Can you work these out from the drawing? Everything is in mm from the part's minimum corner. Give positions to 0.01 mm unless a question says otherwise; leave off trailing zeros. Order: outer loops, then holes, each group sorted by start corner. A loop starts at its lowest first (then second) coordinate and runs counter-clockwise, first axis right, second up. Notation, with made-up numbers: M -27,62 L 11,62 A3 cw 11,66 Z; hole C 63,3.5 d3. An arc over 180 degrees is marked long. Answer as a JSON object with one key per item and string values.
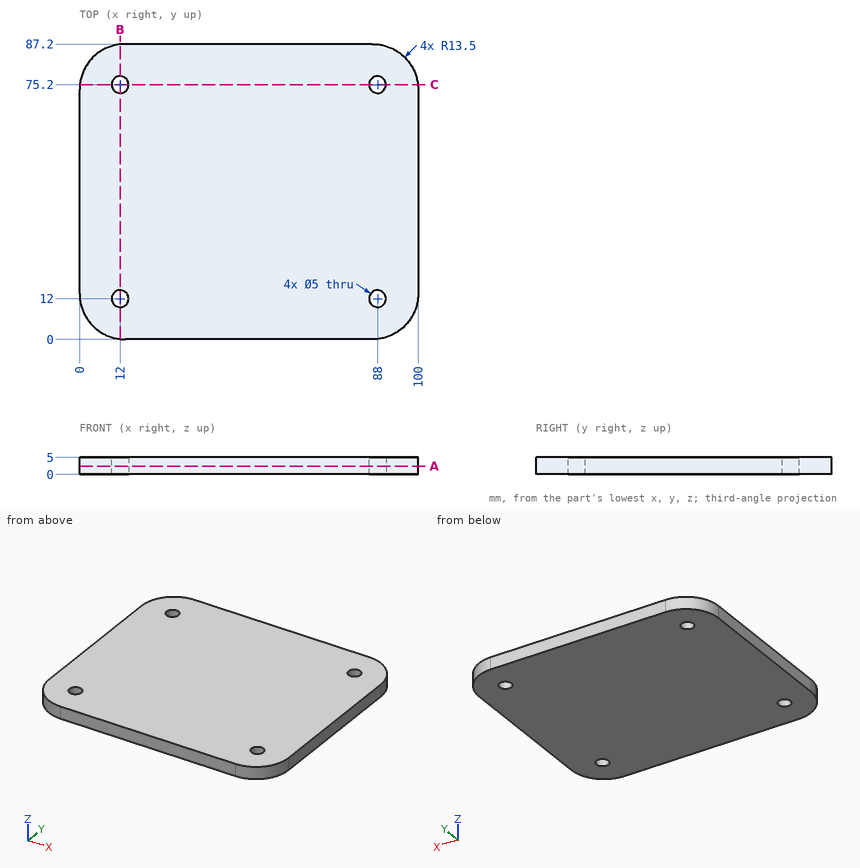
1) I'm going to push a flat-ended pin straight in: pin 1 Ø4 at (x, y) = (88, 75.2) entering from +Z. Where does the tip first touch, or does it pass through?
Results found:
{"pin 1": "passes through"}
2) I want a section at A-A on z = 2.4. Write out the boundary of the cut face in (x, y).
Results found:
{"outline": "M 0,13.5 A13.5 ccw 13.5,0 L 86.5,0 A13.5 ccw 100,13.5 L 100,73.7 A13.5 ccw 86.5,87.2 L 13.5,87.2 A13.5 ccw 0,73.7 Z; hole C 12,12 d5; hole C 12,75.2 d5; hole C 88,12 d5; hole C 88,75.2 d5"}
3) I want a section at C-C on y = 75.2. Write out the boundary of the cut face in (x, z).
Results found:
{"outline": "M 0.08,0 L 9.5,0 L 9.5,5 L 0.08,5 Z; M 14.5,0 L 85.5,0 L 85.5,5 L 14.5,5 Z; M 90.5,0 L 99.92,0 L 99.92,5 L 90.5,5 Z"}
4) I need wall thicknesses on L1, parallel to Y at x = 12, z = 3; L2, parallel to X at y = 77.5, z = 3.75; L3, parallel to Y at x = 96, z = 2.8. Which ranges of each line are inside material? Lowest first, please.
Results found:
{"L1": "y = 0.08 to 9.5, 14.5 to 72.7, 77.7 to 87.12", "L2": "x = 0.55 to 11.02, 12.98 to 87.02, 88.98 to 99.45", "L3": "y = 3.91 to 83.29"}
5) I want a section at B-B on x = 12. Write out the boundary of the cut face in (y, z).
Results found:
{"outline": "M 0.08,0 L 9.5,0 L 9.5,5 L 0.08,5 Z; M 14.5,0 L 72.7,0 L 72.7,5 L 14.5,5 Z; M 77.7,0 L 87.12,0 L 87.12,5 L 77.7,5 Z"}
